Source: CAD feature listing. Evaluate the final solid. Frame: model axes, mm. A direction names the side the tool comes from. Round coordinates to 2 decimals unless told otherwise and drop trailing zeros. Order: outer loops, then holes, each group sorted by start corner. A loop starts at its lowest first (then second) coordinate and runs counter-clockwise, first axis right, second up. Notation, with made-up numbers: (35, 10.25) -> (92, 10.25) arc R28 cw to (92, 39.25) -> close; hole circle Ø10 at (13.25, 20). An arc over 180 degrees is marked (long way). Answer as CSV lines item,"result". Start each with the question number.
(1) Section query B-B (z = -14). Output: boundary loops of the cut face in (x, y).
(2) Section query A-A (x = 14). Output: boundary loops of the cut face in (y, z), plus the area to 3 significant figures.
(3) Pull-direction query (Z, two-part tool) for faces 3 (the cylindrical face through (12.5, 17.75, -14.07)), 4 (the flat face through (0, 17, 19)), 5 (the cylindrical face through (-15.5, 17.75, -14.07)), 6 (the flat face through (-19, 17, 0)); classes: +Z half, -Z half, draft (parallel to the pull), parting line (faces both ways), or undercut.
(4) Section query C-C (y = 29). Output: boundary loops of the cut face in (x, z), plus the area to 3 significant figures.
(5) Section query D-D (x = 0). Output: boundary loops of the cut face in (y, z), plus the area to 3 significant figures.
(6) Line query: line 1 along X through (y, z) = (20.5, -14); line 2 along Z through (x, y) = (-14.5, 14). Output: solid intervals per line, ascending. Write a range as from..to.
(7) Contact query for flat-ended pins moving along their axis: P1, Ø1, axis at x = 6, y = 37.5, coming from the -Z side; P2, Ø10, axis at x = -10, z = -3, coming from the -Y side. Output: stop coordinate, or through.
(8) Set-up query: faces 1 (the cylindrical face through (-1.172, 42.395, -8.923)), 2 (the flat face through (0, 0, 0)). Return all of +Z, -Z, +X, -X, +Y, -Y with unobstructed straight access to the full face (end or side cutting, diameter ignored); none if empty.
```python
from build123d import *

# Parameters (mm, degrees)
SKETCH1_W             = 38
SKETCH1_H             = 38
BOSS_EXTRUDE1_DEPTH   = 35
SKETCH2_R             = 9
BOSS_EXTRUDE2_DEPTH   = 15
F_3_0MM_DOWEL_HOLE1_D = 3


with BuildPart() as part:
    # Sketch1 → Boss-Extrude1 (new body)
    with BuildSketch(Plane(origin=(0, 0, 0), x_dir=(1, 0, 0), z_dir=(0, 1, 0))):
        Rectangle(SKETCH1_W, SKETCH1_H)
    extrude(amount=BOSS_EXTRUDE1_DEPTH)

    # Sketch2 → Boss-Extrude2 (add)
    with BuildSketch(Plane(origin=(0, 35, 0), x_dir=(1, 0, 0), z_dir=(0, 1, 0))):
        Circle(SKETCH2_R)
    extrude(amount=BOSS_EXTRUDE2_DEPTH)

    # Ø3.0mm Dowel Hole1 (through all)
    with Locations(Plane(origin=(0, 0, 0), x_dir=(-1, 0, 0), z_dir=(0, -1, 0))):
        with Locations((-14, -14), (-14, 14), (14, 14), (14, -14)):
            Hole(F_3_0MM_DOWEL_HOLE1_D / 2)


solid = part.part
```
Answer block:
1,outline,"(-19, 0) -> (-15.5, 0) -> (-15.5, 35) -> (-19, 35) -> close; (-12.5, 0) -> (12.5, 0) -> (12.5, 35) -> (-12.5, 35) -> close; (15.5, 0) -> (19, 0) -> (19, 35) -> (15.5, 35) -> close"
2,outline,"(0, -19) -> (35, -19) -> (35, -15.5) -> (0, -15.5) -> close; (0, -12.5) -> (35, -12.5) -> (35, 12.5) -> (0, 12.5) -> close; (0, 15.5) -> (35, 15.5) -> (35, 19) -> (0, 19) -> close"
2,area,"1,120 mm2"
3,face 3,"undercut"
3,face 4,"+Z half"
3,face 5,"undercut"
3,face 6,"draft"
4,outline,"(-19, -19) -> (19, -19) -> (19, 19) -> (-19, 19) -> close; hole circle Ø3 at (-14, -14); hole circle Ø3 at (-14, 14); hole circle Ø3 at (14, -14); hole circle Ø3 at (14, 14)"
4,area,"1,420 mm2"
5,outline,"(0, -19) -> (35, -19) -> (35, -9) -> (50, -9) -> (50, 9) -> (35, 9) -> (35, 19) -> (0, 19) -> close"
5,area,"1,600 mm2"
6,line 1,"-19..-15.5, -12.5..12.5, 15.5..19"
6,line 2,"-19..-15.41, -12.59..12.59, 15.41..19"
7,P1,"z = -7.12"
7,P2,"y = 0"
8,face 1,"+Y"
8,face 2,"+Z, -Z, +X, -X, -Y"
